from build123d import *

# Parameters (mm, degrees)
BOSS_EXTRUDE1_START = 1.5
SKETCH2_R           = 2.75
SKETCH2_R_2         = 20
BOSS_EXTRUDE1_DEPTH = 1.5
FILLET1_R           = 3


with BuildPart() as part:
    # Sketch1 → Revolve1 (revolve)
    with BuildSketch(Plane.XY, mode=Mode.PRIVATE) as revolve1_sk:
        with BuildLine():
            ThreePointArc((0, 30), (-12.5, 17.5), (0, 5))
            Line((0, 5), (0, 30))
        make_face()
        with BuildLine():
            Line((0, 30), (0, 5))
            ThreePointArc((0, 5), (8.838834765, 8.661165235), (12.5, 17.5))
            ThreePointArc((12.5, 17.5), (11.858541226, 21.452847075), (10, 25))
            ThreePointArc((10, 25), (5.590169944, 28.680339887), (0, 30))
        make_face()
        with BuildLine():
            Line((0, 5), (0, 0))
            Line((0, 0), (20, 0))
            Line((20, 0), (20, 12))
            Line((20, 12), (12, 25.5))
            Line((12, 25.5), (10, 25.5))
            Line((10, 25.5), (10, 25))
            ThreePointArc((10, 25), (11.858541226, 21.452847075), (12.5, 17.5))
            ThreePointArc((12.5, 17.5), (8.838834765, 8.661165235), (0, 5))
        make_face()
    revolve(revolve1_sk.sketch.rotate(Axis((0, 0, 0), (0, 1, 0)), 90), axis=Axis((0, 0, 0), (0, 1, 0)))

    # Sketch2 → Boss-Extrude1 (add)
    with BuildSketch(Plane(origin=(0, 0, 0), x_dir=(1, 0, 0), z_dir=(0, 1, 0)).offset(BOSS_EXTRUDE1_START)):
        with BuildLine():
            Line((-11.378629516, 33.382634205), (-20.703132213, 7.441795252))
            ThreePointArc((-20.703132213, 7.441795252), (0, -22), (20.703132213, 7.441795252))
            Line((20.703132213, 7.441795252), (11.378629516, 33.382634205))
            ThreePointArc((11.378629516, 33.382634205), (7.720230047, 38.180047129), (1.968114874, 40))
            Line((1.968114874, 40), (-1.968114874, 40))
            ThreePointArc((-1.968114874, 40), (-7.720230047, 38.180047129), (-11.378629516, 33.382634205))
        make_face()
        with Locations(Location((0, 32, 0), (0, 0, 270))):
            Circle(SKETCH2_R, mode=Mode.SUBTRACT)
        with Locations(Location((0, 0, 0), (0, 0, 90))):
            Circle(SKETCH2_R_2, mode=Mode.SUBTRACT)
    boss_extrude1 = extrude(amount=-BOSS_EXTRUDE1_DEPTH)

    # Mirror1: Boss-Extrude1 across plane
    add(boss_extrude1.mirror(Plane.XY))

    # Fillet1
    fillet1_edges = [part.edges().sort_by_distance(p)[0] for p in [
        (0, 1.5, 20),
    ]]
    fillet(fillet1_edges, radius=FILLET1_R)


solid = part.part
CAD build for the part. Positions are in the model's coordinates, mm. A direction names the side the tool comes from. Round coordinates to 2 decimals unless told otherwise and drop trailing zeros. Loops run counter-clockwise (first coordinate to the right, second up) from the corner with the lowest first, then second, coordinate; pieces in that order, holes last.
(1) Cut at A-A (x = 0). Give the cut face in (y, z).
(2) Cut at C-C (y = 9). Give the cut face in (x, z).
(3) Cut at D-D (y = 17). Give the cut face in (x, z).
(4) Two-plate mould, pull along X, no slides. Class faces 3 (the cylindrical face through (0.121, 0.76, 34.747)), 4 (the flat face through (0, 0, 1)), 5 (the cylindrical face through (22, 1, 0)): +X half, -X half, draft (parallel to the pull), parting line (faces both ways), or undercut.
(5) Cut at B-B (z = -32). Give the cut face in (x, y), plus the area to 3 significant figures.
(6) Which spindle directions (+Z, -Z, +X, -X, +Y, -Y) get a long thin tool onto all of the face, cutting with end or side? Do faces 1 (the cylindrical face through (-0.88, 8.22, 19.98)), 2 (the cylindrical face through (7.79, 0.76, 38.13)). Say none if no direction does.
(7) Drop flat-ended pins along their axis: pin 1 (3.5 mm diameter, centred on x = 0, z = -32, fed in from -Y); pin 2 (5 mm diameter, centred on x = 1, y = 5.5, fed in from +Z); pin 3 (1.5 mm diameter, centred on x = -12.5, y = 14, fed in from -Z); pin 4 (1.5 mm diameter, centred on x = 1, y = 24, fed in from -Z). Give the stop position or say it passes through.
(8) Wall check: line 1 along X through (y, z) = (25.35, 0); line 2 along X through (y, z) = (25.2, 0); line 3 along Y through (x, z) = (4, 27.5). Give the ranges that are in metal, low to high.
Findings below:
1. outline: (0, -40) - (1.5, -40) - (1.5, -34.75) - (0, -34.75) - close; (0, -29.25) - (1.5, -29.25) - (1.5, -23) arc R3 cw to (4.5, -20) - (12, -20) - (25.5, -12) - (25.5, -10) - (25, -10) arc R12.5 ccw to (25, 10) - (25.5, 10) - (25.5, 12) - (12, 20) - (4.5, 20) arc R3 cw to (1.5, 23) - (1.5, 29.25) - (0, 29.25) - close; (0, 34.75) - (1.5, 34.75) - (1.5, 40) - (0, 40) - close
2. outline: circle Ø40 at (0, 0)
3. outline: circle Ø34.07 at (0, 0)
4. face 3: undercut
4. face 4: draft
4. face 5: +X half
5. outline: (-11.88, 0) - (-2.75, 0) - (-2.75, 1.5) - (-11.88, 1.5) - close; (2.75, 0) - (11.88, 0) - (11.88, 1.5) - (2.75, 1.5) - close
5. area: 27.4 mm2
6. face 1: +Y
6. face 2: +Z, +X, +Y, -Y
7. pin 1: passes through
7. pin 2: stops at z = 20.38
7. pin 3: stops at z = -14.92
7. pin 4: stops at z = -13.3
8. line 1: x = -12.09 to -10, -9.73 to 9.73, 10 to 12.09
8. line 2: x = -12.18 to -10, -9.85 to 9.85, 10 to 12.18
8. line 3: y = 0 to 1.5
